Model file for the job. Use its own axes, mm. Give positions to 0.01 mm unless a question says otherwise; leave off trailing zeros. Loops run counter-clockwise (first coordinate to the right, second up) from the corner with the lowest first, then second, coordinate; pieces in that order, holes last. Notation, with made-up numbers: M 21.25,71 L 57.25,71 A31 cw 57.25,107 Z; hole C 67.25,-12.5 d6. An arc over 180 degrees is marked long. Answer in a Markdown table with one row per item.
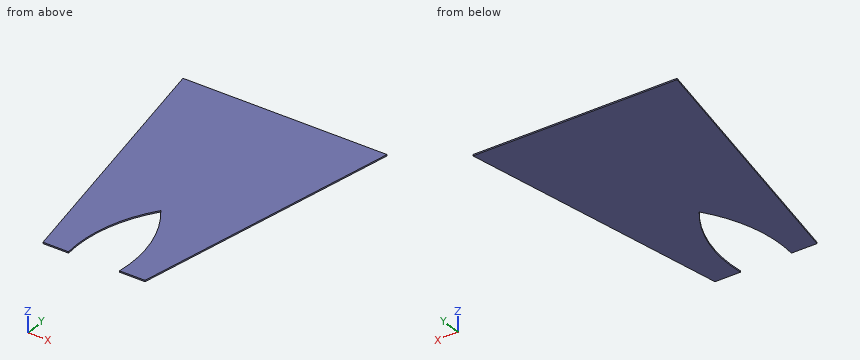
```python
from build123d import *

# Parameters (mm, degrees)
F1_DEPTH = 4


with BuildPart() as f1:
    # F0 (on Top) → F1 (new body)
    with BuildSketch(Plane.XY):
        with BuildLine():
            ThreePointArc((0, 280), (63.755767, 147.032795), (75, 0))
            Line((75, 0), (150, 0))
            Line((150, 0), (300, 800))
            Line((300, 800), (-300, 800))
            Line((-300, 800), (-150, 0))
            Line((-150, 0), (-75, 0))
            ThreePointArc((-75, 0), (-63.755767, 147.032795), (0, 280))
        make_face()
    extrude(amount=F1_DEPTH)


solid = f1.part
```
Q1. Saw through at D-D (y = 262). Give the cut face in (x, z) (3 decimals), and give its area (3 significant figures).
Reported:
| item | result |
|---|---|
| outline | M -199.125,0 L -12.45,0 L -12.45,4 L -199.125,4 Z; M 12.45,0 L 199.125,0 L 199.125,4 L 12.45,4 Z |
| area | 1,490 mm² |
Q2. Saw through at A-A (z = 1.45). Give the cut face in (x, y).
Reported:
| item | result |
|---|---|
| outline | M -300,800 L -150,0 L -75,0 A400 cw 0,280 A400 cw 75,0 L 150,0 L 300,800 Z |
Q3. Saw through at B-B (y = 93.5). Give the cut face in (x, z), and give its area (3 significant figures).
Reported:
| item | result |
|---|---|
| outline | M -167.53,0 L -74.24,0 L -74.24,4 L -167.53,4 Z; M 74.24,0 L 167.53,0 L 167.53,4 L 74.24,4 Z |
| area | 746 mm² |
Q4. Saw through at C-C (x = -225). Give the cut face in (y, z).
Reported:
| item | result |
|---|---|
| outline | M 400,0 L 800,0 L 800,4 L 400,4 Z |
Q5. Probe probe 1 along X at (y, z) = (187, 0.4); probe 2 along X at (y, z) = (189.5, 0.5); probe 3 along X at (y, z) = (324, 3.75). List the from-to ranges inside material, lowest first.
Reported:
| item | result |
|---|---|
| probe 1 | -185.06 to -50.76, 50.76 to 185.06 |
| probe 2 | -185.53 to -49.79, 49.79 to 185.53 |
| probe 3 | -210.75 to 210.75 |
Q6. Drop a flat-ended pin along its axis: pin 1 (5 mm diameter, centred on x = -133, y = 158.5, fed in from -Z). Give the stop position or say it passes through.
Reported:
| item | result |
|---|---|
| pin 1 | z = 0 |
